Read the model definition and answer for the solid it produces. Units are mm, in the model's axes. A direction names the side the tool comes from. Give positions to 0.01 mm unless a question says otherwise; leave off trailing zeros. Order: outer loops, then holes, each group sorted by start corner. A loop starts at its lowest first (then second) coordinate and runs counter-clockwise, first axis right, second up. Notation, with made-up numbers: (2.25, 6.25) - (27.25, 6.25) arc R24 cw to (27.25, 43.25) - close; hole circle Ø9 at (30, 12). An arc over 180 degrees is marked (long way). Use a Markdown table: item, result. Add a question column.
1. A cutting plane is placed at A-A on z = 0. Determine the outline of the cut face in (x, y).
2. A cutting plane is placed at D-D on x = -19. Determine the outline of the cut face in (y, z), and give its area (3 significant figures).
3. Consider L1, parallel to Y at x = -5.5, z = 0; L2, parallel to Y at x = -6, z = -10; L3, parallel to Y at x = -46, z = 3.5. Determine where each line is inside the solid, lowest interval first.
4. Which of the six approach directions +Z, -Z, +X, -X, +Y, -Y give full straight-line access (tool end or side, diameter ignored) to faces 4 (the flat face through (0, 7, 0)), 5 (the flat face through (-27.94, -4, 7)), 6 (the cylindrical face through (-3.57, 4.9, 12.85))?
5. Flat-ended cylindrical pins translate along their axes: P1, Ø10, axis at x = -23.5, z = 7.5, coming from the -Y side; P2, Ø10, axis at x = -40.5, z = -0.5, coming from the +Y side; P3, Ø3, axis at x = -22, z = 1, coming from the +Y side. Find the tip coordinate at first contact, or state that the pin passes through.
6. A cutting plane is placed at C-C on x = -2.5. Determine the outline of the cut face in (y, z), and give its area (3 significant figures).
7. For a pull along Z with two mould halves and no side action, classify faces 1 (the cylindrical face through (-3.67, -5.074, 16.111)), 2 (the flat face through (-7.239, 7.3, 7.3)), 3 (the cylindrical face through (-3.569, 6.088, -9.597)) as released by +Z, released by -Z, zero draft, split by the parting line, or undercut.
8. A cutting plane is placed at B-B on y = 0. Determine the outline of the cut face in (x, z).
```python
from build123d import *

# Parameters (mm, degrees)
SKETCH2_R         = 2.1844
EXTRUDE1_DEPTH    = 57.136011276
CIRPATTERN1_COUNT = 6
SKETCH3_R         = 10.16
SKETCH3_R_2       = 7.261095031
EXTRUDE2_DEPTH    = 22.86


with BuildPart() as part:
    # Sketch1 → Revolve1 (revolve)
    with BuildSketch(Plane.XY, mode=Mode.PRIVATE) as revolve1_sk:
        Polygon((31.75, 0), (31.75, 1.1938), (22.352, 1.1938), (22.352, 6.35), (0, 6.35), (0, 16.891), (-7.239, 16.891), (-7.239, 10.16), (-50.8, 10.16), (-50.8, 0), align=None)
    revolve(revolve1_sk.sketch.rotate(Axis((-40.728426743, 0, 0), (1, 0, 0)), 90), axis=Axis((-40.728426743, 0, 0), (1, 0, 0)))

    # Sketch2 → Extrude1 (cut, through all)
    with BuildSketch(Plane(origin=(0, 0, 0), x_dir=(0, 0, -1), z_dir=(1, 0, 0))):
        with Locations((0, 13.4874)):
            Circle(SKETCH2_R)
    extrude1 = extrude(amount=-EXTRUDE1_DEPTH, mode=Mode.SUBTRACT)

    # CirPattern1: Extrude1 ×6 about axis
    cirpattern1_axis = Axis((0, 0, 0), (1, 0, 0))
    for i in range(1, CIRPATTERN1_COUNT):
        add(extrude1.rotate(cirpattern1_axis, i * 360 / CIRPATTERN1_COUNT), mode=Mode.SUBTRACT)

    # Sketch3 → Extrude2 (cut)
    with BuildSketch(Plane.ZY.offset(50.8)):
        Circle(SKETCH3_R)
        Circle(SKETCH3_R_2, mode=Mode.SUBTRACT)
    extrude(amount=-EXTRUDE2_DEPTH, mode=Mode.SUBTRACT)


solid = part.part
```
Output values:
| question | item | result |
|---|---|---|
| 1 | outline | (-50.8, -7.26) - (-27.94, -7.26) - (-27.94, -10.16) - (-7.24, -10.16) - (-7.24, -11.3) - (0, -11.3) - (0, -6.35) - (22.35, -6.35) - (22.35, -1.19) - (31.75, -1.19) - (31.75, 1.19) - (22.35, 1.19) - (22.35, 6.35) - (0, 6.35) - (0, 11.3) - (-7.24, 11.3) - (-7.24, 10.16) - (-27.94, 10.16) - (-27.94, 7.26) - (-50.8, 7.26) - close; (-7.24, -16.89) - (0, -16.89) - (0, -15.67) - (-7.24, -15.67) - close; (-7.24, 15.67) - (0, 15.67) - (0, 16.89) - (-7.24, 16.89) - close |
| 2 | outline | circle Ø20.32 at (0, 0) |
| 2 | area | 324 mm² |
| 3 | L1 | -16.89 to -15.67, -11.3 to 11.3, 15.67 to 16.89 |
| 3 | L2 | -13.61 to -8.14, -5.35 to 5.35, 8.14 to 13.61 |
| 3 | L3 | -6.36 to 6.36 |
| 4 | face 4 | +X |
| 4 | face 5 | -X |
| 4 | face 6 | +X, -X |
| 5 | P1 | y = -9.85 |
| 5 | P2 | y = 7.26 |
| 5 | P3 | y = 10.16 |
| 6 | outline | circle Ø33.78 at (0, 0); hole circle Ø4.37 at (-13.49, 0); hole circle Ø4.37 at (-6.74, -11.68); hole circle Ø4.37 at (-6.74, 11.68); hole circle Ø4.37 at (6.74, -11.68); hole circle Ø4.37 at (6.74, 11.68); hole circle Ø4.37 at (13.49, 0) |
| 6 | area | 806 mm² |
| 7 | face 1 | split by the parting line |
| 7 | face 2 | zero draft |
| 7 | face 3 | undercut |
| 8 | outline | (-50.8, -7.26) - (-27.94, -7.26) - (-27.94, -10.16) - (-7.24, -10.16) - (-7.24, -16.89) - (0, -16.89) - (0, -6.35) - (22.35, -6.35) - (22.35, -1.19) - (31.75, -1.19) - (31.75, 1.19) - (22.35, 1.19) - (22.35, 6.35) - (0, 6.35) - (0, 16.89) - (-7.24, 16.89) - (-7.24, 10.16) - (-27.94, 10.16) - (-27.94, 7.26) - (-50.8, 7.26) - close |
